```python
from build123d import *

# Parameters (mm, degrees)
F0_R      = 12.7
F0_W      = 19.2045877871
F0_H      = 34.798
F1_DEPTH  = 60.325
F2_W      = 54.1596032441
F2_H      = 22.3266
F3_DEPTH  = 34.799
F4_W      = 44.103635475
F4_H      = 22.1672710031
F5_DEPTH  = 25.4
F6_DEPTH  = 19.05
F7_DEPTH  = 19.05
F8_W      = 41.275
F8_H      = 34.798
F9_DEPTH  = 50.8
F10_R     = 6.35
F11_DEPTH = 22.226
F12_R     = 5.08


with BuildPart() as f1:
    # F0 (on Front) → F1 (new body)
    with BuildSketch(Plane.XZ):
        with BuildLine():
            Line((85.852, 0), (22.225, 0))
            ThreePointArc((22.225, 0), (15.7154482119, -15.7154482119), (0, -22.225))
            Line((0, -22.225), (91.694, -22.225))
            Line((91.694, -22.225), (85.852, 0))
        make_face()
        with BuildLine():
            ThreePointArc((0, -22.225), (15.7154482119, -15.7154482119), (22.225, 0))
            ThreePointArc((22.225, 0), (-15.7154482119, 15.7154482119), (0, -22.225))
        make_face()
        Circle(F0_R, mode=Mode.SUBTRACT)
        Polygon((130.8840122129, 0), (117.094, 0), (117.094, -22.225), (194.2084, -22.225), (194.2084, 0), (150.0886, 0), align=None)
        Polygon((117.094, 0), (85.852, 0), (91.694, -22.225), (117.094, -22.225), align=None)
        with BuildLine():
            ThreePointArc((130.8840122129, 34.798), (127.3108445203, 16.0825969798), (117.094, 0))
            Line((117.094, 0), (130.8840122129, 0))
            Line((130.8840122129, 0), (130.8840122129, 34.798))
        make_face()
        with Locations((140.4863061065, 17.399)):
            Rectangle(F0_W, F0_H)
    extrude(amount=F1_DEPTH)

    # F2 (on Top) → F3 (cut, through all)
    with BuildSketch(Plane.XY):
        with Locations((0.2378355712, -30.1625)):
            Rectangle(F2_W, F2_H)
    extrude(amount=F3_DEPTH, mode=Mode.SUBTRACT)

    # F4 (on Top) → F5 (cut)
    with BuildSketch(Plane.XY):
        with Locations((-0.2239840105, -30.3645441309)):
            Rectangle(F4_W, F4_H)
    extrude(amount=-F5_DEPTH, mode=Mode.SUBTRACT)

    # F0 (on Front) → F6 (cut)
    with BuildSketch(Plane.XZ):
        Polygon((117.094, 0), (85.852, 0), (91.694, -22.225), (117.094, -22.225), align=None)
    extrude(amount=-F6_DEPTH, mode=Mode.SUBTRACT)

    # F0 (on Front) → F7 (cut)
    with BuildSketch(Plane.XZ):
        Polygon((117.094, 0), (85.852, 0), (91.694, -22.225), (117.094, -22.225), align=None)
    extrude(amount=F7_DEPTH, mode=Mode.SUBTRACT)

    # F8 (on face) → F9 (cut)
    with BuildSketch(Plane.YZ.offset(150.0886)):
        with Locations((-39.6875, 17.399)):
            Rectangle(F8_W, F8_H)
    extrude(amount=-F9_DEPTH, mode=Mode.SUBTRACT)

    # F10 (on face) → F11 (cut, through all)
    with BuildSketch(Plane.XY):
        with Locations((155.3464, -31.623)):
            Circle(F10_R)
    extrude(amount=-F11_DEPTH, mode=Mode.SUBTRACT)

    # F12
    f12_edges = [f1.edges().sort_by_distance(p)[0] for p in [
        (150.0886, -9.525, 34.798),
        (150.0886, -9.525, 0),
        (194.2084, -30.1625, 0),
        (22.225, -50.8254, 0),
        (22.225, -9.4996, 0),
    ]]
    fillet(f12_edges, radius=F12_R)


solid = f1.part
```
Design review of the part built by this model. Coordinates are the model's own, in mm. A direction names the side the tool comes from. Coordinates: 2 decimals unless noted, no trailing zeros. Loops run counter-clockwise (first coordinate to the right, second up) from the corner with the lowest first, then second, coordinate; pieces in that order, holes last. Notation, with made-up numbers: (53, 64.25) - (106, 64.25) arc R22 ccw to (106, 88.25) - close; hole circle Ø5 at (74, 26.5). An arc over 180 degrees is marked (long way). Use CSV: the item, a comma, the result in double quotes. Start each with the question number.
1) Consider section C-C on z = -16. Write out the cut boundary in (x, y) (3 decimals), then the cut area to 3 significant figures.
2) Consider section D-D on z = 17. Write out the cut boundary in (x, y) (3 decimals), then the cut area to 3 significant figures.
3) For pin 1 Ø21 at (y, z) = (-10.5, 18) entering from +X; pin 2 Ø6.5 at (x, z) = (99, -7) entering from +Y; pin 3 Ø1 at (y, z) = (-11.5, 11.5) entering from -X, all flat-tipped, find the tip position at first contact; note any pin that passes through.
4) The part is to be moulded in two halves that separate along Y. For faces 1 (the flat face through (138, -9, 34.798)), 2 (the flat face through (2, -18.999, 13)), 3 (the flat face through (101, -19.05, -11)), 4 (the cylindrical face through (161.4, -29.7, -11)), say which applies: +Y half, -Y half, draft (parallel to the pull), parting line (faces both ways), or undercut.
5) Tool access review of faces 5 (the flat face through (88.732, -9.392, -10.957)), 6 (the flat face through (136, -19.05, 17)), 7 (the flat face through (117.094, -9, -11)), 8 (the cylindrical face through (23.55, -9.63, 1.2)): name each direction out of +Z, -Z, +X, -X, +Y, -Y from which nothing blocks a thin tool from reaching the whole face with its end or side.
6) Consider section A-A on y = -13.5. Write out the cut boundary in (x, z) (3 decimals).
7) Consider section B-B on z = 7. Write out the cut boundary in (x, y) (3 decimals), then the cut area to 3 significant figures.
8) Wall thickness on L1, parallel to X at y = -18.5, z = -3.5; L2, parallel to Y at x = 12.5, z = -19 (3 decimals); L3, parallel to Z at x = 0, y = -9 (3 decimals): over which ranges is each line inside the solid? List them lowest first. Write a range as from..to.
Geometry says:
1,outline,"(-15.426, -60.325) - (194.208, -60.325) - (194.208, 0) - (117.094, 0) - (117.094, -19.05) - (90.058, -19.05) - (90.058, 0) - (-15.426, 0) - (-15.426, -19.281) - (21.828, -19.281) - (21.828, -41.448) - (-15.426, -41.448) - close; hole circle Ø12.7 at (155.346, -31.623)"
1,area,"11,200 mm^2"
2,outline,"(-14.316, -60.325) - (14.316, -60.325) - (14.316, -41.326) - (-14.316, -41.326) - close; (-14.316, -18.999) - (14.316, -18.999) - (14.316, 0) - (-14.316, 0) - close; (127.664, -19.05) - (150.089, -19.05) - (150.089, 0) - (127.664, 0) - close"
2,area,"1,520 mm^2"
3,pin 1,"x = 150.09"
3,pin 2,"y = -19.05"
3,pin 3,"x = -19.31"
4,face 1,"draft"
4,face 2,"undercut"
4,face 3,"+Y half"
4,face 4,"undercut"
5,face 5,"+Z, +Y"
5,face 6,"+Z, +X, -X, -Y"
5,face 7,"+Z, -Z, +Y"
5,face 8,"+Z, +Y, -Y"
6,outline,"(0, -22.225) - (91.694, -22.225) - (85.852, 0) - (26.828, 0) arc R5.08 cw to (21.837, 4.135) arc R22.225 ccw (long way) to start; (117.094, -22.225) - (194.208, -22.225) - (194.208, -5.08) arc R5.08 ccw to (189.128, 0) - (155.169, 0) arc R5.08 cw to (150.089, 5.08) - (150.089, 29.718) arc R5.08 ccw to (145.009, 34.798) - (130.884, 34.798) arc R50.8 cw to (117.094, 0) - close; hole circle Ø25.4 at (0, 0)"
7,outline,"(-21.094, -60.325) - (-10.597, -60.325) - (-10.597, -41.326) - (-21.094, -41.326) - close; (-21.094, -18.999) - (-10.597, -18.999) - (-10.597, 0) - (-21.094, 0) - close; (10.597, -60.325) - (21.094, -60.325) - (21.094, -41.326) - (10.597, -41.326) - close; (10.597, -18.999) - (21.094, -18.999) - (21.094, 0) - (10.597, 0) - close; (122.604, -19.05) - (150.089, -19.05) - (150.089, 0) - (122.604, 0) - close"
7,area,"1,320 mm^2"
8,L1,"-21.95..-12.21, 12.21..86.77, 117.09..193.96"
8,L2,"-60.325..-41.448, -19.281..0"
8,L3,"-22.225..-12.7, 12.7..22.225"
